The listing builds one solid part. Answer for the finished solid, in the listing's coordinates (mm). A direction names the side the tool comes from. Coordinates: 2 decimals unless noted, no trailing zeros. Loops run counter-clockwise (first coordinate to the right, second up) from the corner with the lowest first, then second, coordinate; pieces in that order, holes last. Notation, with made-up numbers: (82, -31) -> (118, -31) arc R24 ccw to (118, 4) -> close; hole circle Ø4 at (38.5, -1.5). An arc over 180 degrees is marked (long way). Answer in a Markdown table with one row per item.
```python
from build123d import *

# Parameters (mm, degrees)
F0_W     = 41.625001
F0_H     = 41.625001
F0_W_2   = 29.625001
F0_H_2   = 29.625001
F1_DEPTH = 160
F3_D     = 6


with BuildPart() as f1:
    # F0 (on Right) → F1 (new body)
    with BuildSketch(Plane.YZ):
        with Locations((-20.8125, 20.8125)):
            Rectangle(F0_W, F0_H)
        with Locations((-20.8125, 20.8125)):
            Rectangle(F0_W_2, F0_H_2, mode=Mode.SUBTRACT)
    extrude(amount=F1_DEPTH)

    # F3 (through all)
    with Locations(Plane.XY.offset(41.625001)):
        with Locations((135, -20.8125), (80, -20.8125), (25, -20.8125)):
            Hole(F3_D / 2)


solid = f1.part
```
Item 1: A cutting plane is placed at D-D, the plane x = 45. Determine the outline of the cut face in (y, z) (3 decimals).
Findings below:
| item | result |
|---|---|
| outline | (-41.625, 0) -> (0, 0) -> (0, 41.625) -> (-41.625, 41.625) -> close; hole (-35.625, 6) -> (-6, 6) -> (-6, 35.625) -> (-35.625, 35.625) -> close |
Item 2: Determine the mould class of faces 1 (the face through (0, -40, 21)), 2 (the face through (25.65, -23.74, 38.58)), 3 (the face through (79, -26, 41.625)) for opening direction X: +X half, -X half, draft (parallel to the pull), parting line (faces both ways), or undercut.
Findings below:
| item | result |
|---|---|
| face 1 | -X half |
| face 2 | undercut |
| face 3 | draft |
Item 3: A cutting plane is placed at A-A, the plane z = 21. Determine the outline of the cut face in (x, y) (3 decimals).
Findings below:
| item | result |
|---|---|
| outline | (0, -41.625) -> (160, -41.625) -> (160, -35.625) -> (0, -35.625) -> close; (0, -6) -> (160, -6) -> (160, 0) -> (0, 0) -> close |
Item 4: A tool of negligible diameter and unlimited length cuts with its end or side. For faces 4 (the face through (79, -6, 21)), 5 (the face through (160, -40, 21)), from which of +Z, -Z, +X, -X, +Y, -Y can it reach the whole face along a straight path? Write none if from no direction.
Findings below:
| item | result |
|---|---|
| face 4 | +X, -X |
| face 5 | +Z, -Z, +X, +Y, -Y |
Item 5: Find the intervals of material crossed by probe 1 along Z at (x, y) = (35, -29.5) (3 decimals); probe 2 along Y at (x, z) = (34, 33.5) (3 decimals); probe 3 along Y at (x, z) = (25, 38) (1 decimal), in increasing order.
Findings below:
| item | result |
|---|---|
| probe 1 | z = 0 to 6, 35.625 to 41.625 |
| probe 2 | y = -41.625 to -35.625, -6 to 0 |
| probe 3 | y = -41.6 to -23.8, -17.8 to 0 |
Item 6: A flat-ended cylindrical pin translates along its axis: pin 1 Ø3.5 at (x, y) = (80, -20.81) entering from +Z. Find the tip coordinate at first contact, or state that the pin passes through.
Findings below:
| item | result |
|---|---|
| pin 1 | passes through |
Item 7: A cutting plane is placed at C-C, the plane y = -29. Determine the outline of the cut face in (x, z) (3 decimals), plus the area to 3 significant figures.
Findings below:
| item | result |
|---|---|
| outline | (0, 0) -> (160, 0) -> (160, 6) -> (0, 6) -> close; (0, 35.625) -> (160, 35.625) -> (160, 41.625) -> (0, 41.625) -> close |
| area | 1,920 mm2 |
Item 8: A cutting plane is placed at B-B, the plane x = 135. Determine the outline of the cut face in (y, z) (1 decimal).
Findings below:
| item | result |
|---|---|
| outline | (-41.6, 0) -> (-23.8, 0) -> (-23.8, 6) -> (-35.6, 6) -> (-35.6, 35.6) -> (-23.8, 35.6) -> (-23.8, 41.6) -> (-41.6, 41.6) -> close; (-17.8, 0) -> (0, 0) -> (0, 41.6) -> (-17.8, 41.6) -> (-17.8, 35.6) -> (-6, 35.6) -> (-6, 6) -> (-17.8, 6) -> close |
